Part print with two shaded views. Sizes in mm from the minimum x, y, z corner. A direction names the side the tool comes from. Coordinates: 2 decimals unless noted, no trailing zeros. Write each loop counter-clockwise with the first axis right and the second up, starting at its lowest first coordinate (ties: lowest second). Pieces come first, ordered by that corner, then holes. Notation, with made-up numbers: (-22.5, 64) - (17.5, 64) arc R9 cw to (17.5, 77) - close; hole circle Ø6 at (61.25, 36.5). An arc over 180 degrees is marked (long way). One line per question, with ' | ' between items. Start each with the question number.
1. Probe line 1 (X direction, y = 17.5, z = 21.5); line 2 (Y direction, x = 45, z = 32); line 3 (X direction, y = 19, z = 21). List the from-to ranges inside material, lowest first.
2. Band-saw the part on B-B, the plane z = 32. Write the cut outline in (x, y) (1 decimal).
3. Flat gauge pins, fed straight in: P1, Ø8, axis at y = 16.5, z = 24.5, coming from the +X side; P2, Ø2.5, axis at x = 31, y = 14.5, coming from the -Z side; P3, Ø1, axis at x = 46, z = 37, coming from the +Y side. Where does each tip first touch, or does it go through?
4. Band-saw the part on D-D, the plane z = 19.5. Write the cut outline in (x, y), then the cut area to 3 significant figures.
5. Band-saw the part on C-C, the plane x = 27. Write the cut outline in (y, z).
6. Band-saw the part on A-A, the plane x = 36. Write the cut outline in (y, z).
7. Two-plate mould, pull along Z, no slides. Class the marked faces 4, 5 and 6: +Z half, -Z half, draft (parallel to the pull), parting line (faces both ways), or undercut.
8. Which spindle directions (+Z, -Z, +X, -X, +Y, -Y) get a long thin tool onto all of the face, cutting with end or side? Do the marked faces 1, 2 and 3. Say none if no direction does.
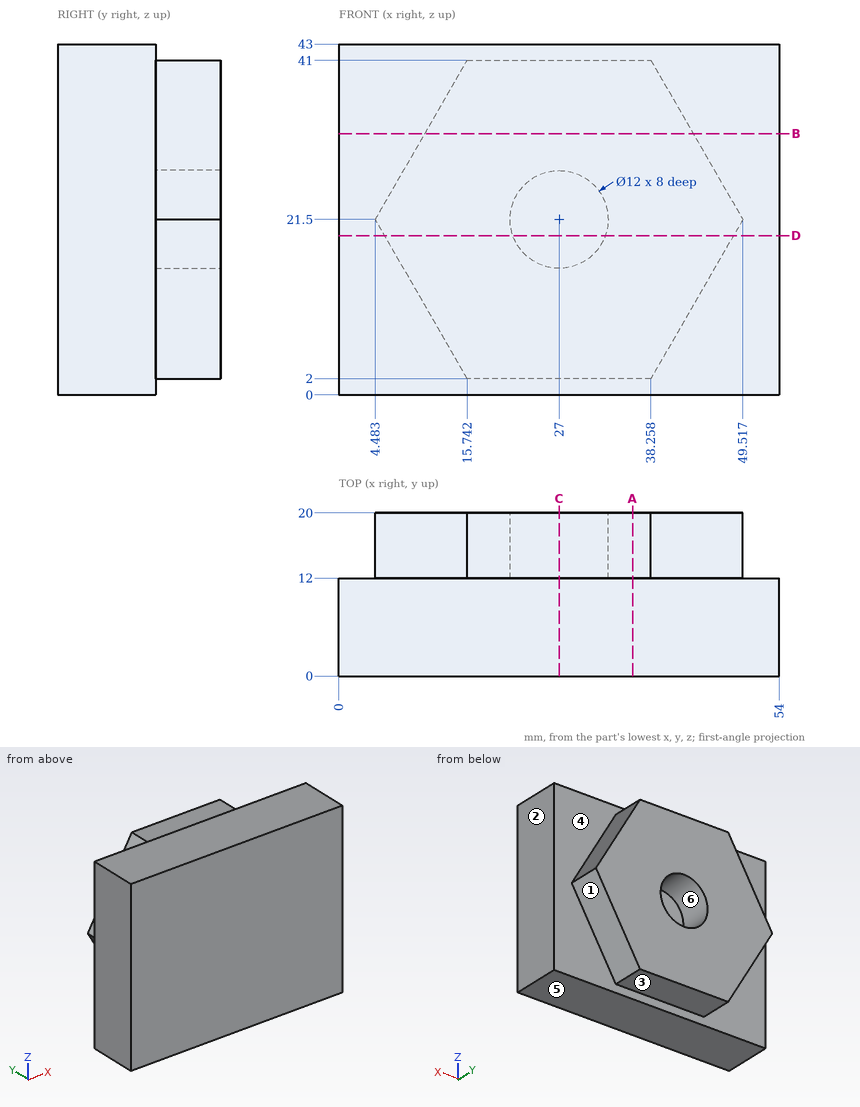
Filled in:
1) line 1: x = 4.48 to 21, 33 to 49.52 | line 2: y = 0 to 12 | line 3: x = 4.77 to 21.02, 32.98 to 49.23
2) outline: (0, 0) - (54, 0) - (54, 12) - (43.5, 12) - (43.5, 20) - (10.5, 20) - (10.5, 12) - (0, 12) - close
3) P1: stops at x = 49.52 | P2: stops at z = 2 | P3: stops at y = 12
4) outline: (0, 0) - (54, 0) - (54, 12) - (48.36, 12) - (48.36, 20) - (32.66, 20) - (32.66, 12) - (21.34, 12) - (21.34, 20) - (5.64, 20) - (5.64, 12) - (0, 12) - close | area: 899 mm²
5) outline: (0, 0) - (12, 0) - (12, 2) - (20, 2) - (20, 15.5) - (12, 15.5) - (12, 27.5) - (20, 27.5) - (20, 41) - (12, 41) - (12, 43) - (0, 43) - close
6) outline: (0, 0) - (12, 0) - (12, 2) - (20, 2) - (20, 41) - (12, 41) - (12, 43) - (0, 43) - close
7) face 4: draft | face 5: -Z half | face 6: undercut
8) face 1: -Z, +X, +Y | face 2: +Z, -Z, +X, +Y, -Y | face 3: -Z, +X, -X, +Y
